Verification items for the finished model (mm, model axes). A direction names the side the tool comes from. Round coordinates to 2 decimals unless told otherwise and drop trailing zeros. Write each loop counter-clockwise with the first axis right and the second up, starting at its lowest first coordinate (ties: lowest second). Pieces come first, ordered by that corner, then holes. Notation, with made-up numbers: (-22.5, 53) - (-12.5, 53) arc R15 cw to (-12.5, 76) - close; hole circle Ø4 at (14.25, 9). An arc over 180 degrees is marked (long way). Answer as a JSON object with one key per item and string values. Group by question number.
1) Set-up check for faces 1 (the cylindrical face through (-17.215, 1.801, 1.521)), 2 (the cylindrical face through (17.331, -4.905, 1.521)): record each of +Z, -Z, +X, -X, +Y, -Y from which the full face is reachable in a straight line by a thin tool's end or side.
2) Thickness scan on line 1 (Y direction, x = -0.5, z = 2.65); line 2 (Y direction, x = 0.5, z = 0.55); line 3 (X direction, y = -0.5, z = 0.55). Record the ranges inside material, lowest first.
3) Mould release check, pull along Y, two halves, no side actions. Record for faces 3 (the flat face through (-8, 1.5, 1)), 4 (the flat face through (-17.5, -3, 1)), 5 (the cylindrical face through (-17.34, -4.89, 1.52)): +Y half, -Y half, draft (parallel to the pull), parting line (faces both ways), or undercut.
4) Section check B-B (z = 2.6). Enter the section's corners in (x, y), then the cut area to 3 significant figures.
5) Section check C-C (y = -0.25). Enter the section's corners in (x, z), then the cut area to 3 significant figures.
6) Go/stop test with flat-tipped pins: pin 1 Ø1.5 at (x, z) = (13, 1.5) entering from -Y; pin 2 Ø1.5 at (x, z) = (-8, 2) entering from +Y; pin 3 Ø1.5 at (x, z) = (3, 1.5) entering from -Y. Record where each tip stops, or that it passes through.
7) Section check D-D (x = -14). Enter the section's corners in (y, z), then the cut area to 3 significant figures.
8) Section check A-A (x = -2). Enter the section's corners in (y, z).
```python
from build123d import *

# Parameters (mm, degrees)
EXTRUDE_1_DEPTH = 3
FILLET_1_R      = 1


with BuildPart() as part:
    # Эскиз1 → Бобышка-Вытянуть1 (new body)
    with BuildSketch(Plane.XY):
        Polygon((-17.5, -1.5), (-17.5, -5), (17.5, -5), (17.5, 5), (-17.5, 5), (-17.5, 1.5), (0, 1.5), (0, -1.5), align=None)
        with BuildLine():
            ThreePointArc((-17.5, 5), (0, 8.770166538), (17.5, 5))
            Line((17.5, 5), (-17.5, 5))
        make_face()
        with BuildLine():
            Line((-17.5, -5), (17.5, -5))
            ThreePointArc((17.5, -5), (0, -8.770166538), (-17.5, -5))
        make_face()
    extrude(amount=EXTRUDE_1_DEPTH)

    # Скругление1
    fillet_1_edges = [part.edges().sort_by_distance(p)[0] for p in [
        (-17.5, 1.5, 1.5),
        (-17.5, 5, 1.5),
        (17.5, 5, 1.5),
        (17.5, -5, 1.5),
        (-17.5, -5, 1.5),
        (-17.5, -1.5, 1.5),
    ]]
    fillet(fillet_1_edges, radius=FILLET_1_R)


solid = part.part
```
Returned:
{
 "1": {"face 1": "+Z, -Z, -X", "face 2": "+Z, -Z, +X, -Y"},
 "2": {"line 1": "-8.77 to -1.5, 1.5 to 8.77", "line 2": "-8.77 to 8.77", "line 3": "0 to 17.5"},
 "3": {"face 3": "undercut", "face 4": "draft", "face 5": "-Y half"},
 "4": {"outline": "(-17.5, -4.35) arc R1 ccw to (-16.9, -5.27) arc R42.5 ccw to (16.9, -5.27) arc R1 ccw to (17.5, -4.35) - (17.5, 4.35) arc R1 ccw to (16.9, 5.27) arc R42.5 ccw to (-16.9, 5.27) arc R1 ccw to (-17.5, 4.35) - (-17.5, 2.5) arc R1 ccw to (-16.5, 1.5) - (0, 1.5) - (0, -1.5) - (-16.5, -1.5) arc R1 ccw to (-17.5, -2.5) - close", "area": "474 mm2"},
 "5": {"outline": "(0, 0) - (17.5, 0) - (17.5, 3) - (0, 3) - close", "area": "52.5 mm2"},
 "6": {"pin 1": "y = -6.97", "pin 2": "y = 8.15", "pin 3": "y = -8.71"},
 "7": {"outline": "(-6.4, 0) - (-1.5, 0) - (-1.5, 3) - (-6.4, 3) - close; (1.5, 0) - (6.4, 0) - (6.4, 3) - (1.5, 3) - close", "area": "29.4 mm2"},
 "8": {"outline": "(-8.72, 0) - (-1.5, 0) - (-1.5, 3) - (-8.72, 3) - close; (1.5, 0) - (8.72, 0) - (8.72, 3) - (1.5, 3) - close"}
}
